Geometry: final body of the model. Coordinates: model frame, mm. A direction names the side the tool comes from. Coordinates: 2 decimals unless noted, no trailing zeros. Order: outer loops, then holes, each group sorted by start corner. A loop starts at its lowest first (then second) coordinate and runs counter-clockwise, first axis right, second up. Notation, with made-up numbers: M 66,-16 L 75,-16 A5 ccw 75,-8 Z; hole C -28.75,66 d9. An arc over 180 degrees is marked long. Use CSV: the item, a comma, the result in double quotes. Start each with the question number.
Q1. Section query C-C, the plane z = -38. Output: boundary loops of the cut face in (x, y), and give its area (3 significant figures).
Q2. Section query B-B, the plane x = 19.5. Output: boundary loops of the cut face in (y, z), and give its area (4 significant figures).
Q3. Mould query, pull axis Z, two halves, no side actions, for faces 1 (the face through (16, 25, -5)), 2 (the face through (-2, 0, -44)), 3 (the face through (10, 16, 50)), 4 (the face through (16, 25, -33)). Classes: +Z half, -Z half, draft (parallel to the pull), parting line (faces both ways), or undercut.
Q4. Section query D-D, the plane y = 3. Output: boundary loops of the cut face in (x, z), and give its area (3 significant figures).
Q5. First-contact query: P1, Ø4.5, axis at x = 9.5, z = 40, coming from the -Y side; P2, Ø0.9, axis at x = 2.5, z = -51.5, coming from the +Y side; P3, Ø7.5, axis at x = 12, y = 28, coming from the -Z side. Flat tips, straight axial feed; report the tip coordinate or a pass-through.
Q6. Access query for faces 5 (the face through (8.92, 25.31, -28.44)), 6 (the face through (12, 5.25, -43)), 7 (the face through (7, 14.75, 0)), 8 (the face through (7, 0.25, -51)), 9 (the face through (12, 7, -51)). Directions: +Z, -Z, +X, -X, +Y, -Y. A direction counts if a zero-diameter tool reaches every point of the face in a straight line with its end or side. Return the directions, or none.
Q7. Ray query, probe 1 along Z at (x, y) = (14.75, 23); probe 2 along Z at (x, y) = (15.5, 13.5); probe 3 along Z at (x, y) = (5.75, 8). Return the intervals inside material, ascending.
Q8. Section query A-A, the plane y = -7. Output: boundary loops of the cut face in (x, z).
from build123d import *

# Parameters (mm, degrees)
BOSS_EXTRUDE1_DEPTH      = 50
BOSS_EXTRUDE1_DEPTH_BACK = 50
CUT_EXTRUDE1_DEPTH       = 66.448930473
CUT_EXTRUDE1_DEPTH_BACK  = 66.448930473
SKETCH2_W                = 70
SKETCH2_H                = 29.5
SKETCH5_W                = 15
SKETCH5_H                = 9
CUT_EXTRUDE2_DEPTH       = 20
BOSS_EXTRUDE3_REACH      = 110.128
BOSS_EXTRUDE4_DEPTH      = 3


with BuildPart() as part:
    # Sketch1 → Boss-Extrude1 (new, two sides: drawn at the far end of the back side and taken through both)
    with BuildSketch(Plane.XY.offset(-BOSS_EXTRUDE1_DEPTH_BACK)):
        with BuildLine():
            Line((-2, -14.75), (2, -14.75))
            Line((2, -14.75), (2, 5.25))
            Line((2, 5.25), (22, 5.25))
            Line((22, 5.25), (22, 14.75))
            Line((22, 14.75), (22, 34.75))
            Line((22, 34.75), (10.449961479, 34.75))
            ThreePointArc((10.449961479, 34.75), (6.111442266, 23.465706156), (-2, 14.501190503))
            Line((-2, 14.501190503), (-2, -14.75))
        make_face()
    extrude(amount=BOSS_EXTRUDE1_DEPTH + BOSS_EXTRUDE1_DEPTH_BACK)

    # Sketch2 → Cut-Extrude1 (cut, two sides: drawn at the far end of the back side and taken through both)
    with BuildSketch(Plane(origin=(-2, 0, 0), x_dir=(0, 0, -1), z_dir=(1, 0, 0)).offset(-CUT_EXTRUDE1_DEPTH_BACK)):
        Rectangle(SKETCH2_W, SKETCH2_H)
    extrude(amount=CUT_EXTRUDE1_DEPTH + CUT_EXTRUDE1_DEPTH_BACK, mode=Mode.SUBTRACT)

    # Sketch5 → Cut-Extrude2 (cut)
    with BuildSketch(Plane(origin=(0, 34.75, 0), x_dir=(1, 0, 0), z_dir=(0, 1, 0))):
        with Locations((14.5, -28.5)):
            Rectangle(SKETCH5_W, SKETCH5_H)
        with Locations((14.5, -9.5)):
            Rectangle(SKETCH5_W, SKETCH5_H)
        with Locations((14.5, 9.5)):
            Rectangle(SKETCH5_W, SKETCH5_H)
        with Locations((14.5, 28.5)):
            Rectangle(SKETCH5_W, SKETCH5_H)
    extrude(amount=-CUT_EXTRUDE2_DEPTH, mode=Mode.SUBTRACT)

    # Boss-Extrude3: up to this face of the body (flat: up to its plane)
    boss_extrude3_end = Plane(part.part.faces().sort_by_distance((10.585369563, 14.996232635, -50))[0])
    # Sketch6 → Boss-Extrude3 (add, up to the picked face)
    with BuildSketch(Plane.XY.offset(50), mode=Mode.PRIVATE) as boss_extrude3_sk1:
        with BuildLine():
            Line((14.639320225, 34.75), (10.449961479, 34.75))
            ThreePointArc((10.449961479, 34.75), (9.109168973, 29.740022443), (7, 25.001984252))
            Line((7, 25.001984252), (7, 14.75))
            ThreePointArc((7, 14.75), (8.974829231, 25.454662693), (14.639320225, 34.75))
        make_face()
    boss_extrude3_tool1 = split(extrude(boss_extrude3_sk1.sketch, amount=-BOSS_EXTRUDE3_REACH, mode=Mode.PRIVATE), bisect_by=boss_extrude3_end, keep=Keep.BOTH, mode=Mode.PRIVATE)
    add(boss_extrude3_tool1.solids().sort_by(Axis((9.906803, 28.936431, 50), (0, 0, -1)))[0])

    # Sketch8 → Boss-Extrude4 (add)
    with BuildSketch(Plane(origin=(0, 0, -50), x_dir=(-1, 0, 0), z_dir=(0, 0, -1))):
        Polygon((-12, 0.25), (-2, 0.25), (-2, -14.75), (2, -14.75), (2, 14.501190503), (-12, 14.501190503), align=None)
    extrude(amount=BOSS_EXTRUDE4_DEPTH)


solid = part.part
Responses:
1,outline,"M -2,-14.75 L 2,-14.75 L 2,5.25 L 22,5.25 L 22,34.75 L 10.45,34.75 A33 cw -2,14.5 Z"
1,area,"627 mm²"
2,outline,"M 5.25,-50 L 34.75,-50 L 34.75,-33 L 14.75,-33 L 14.75,-35 L 5.25,-35 Z; M 5.25,35 L 14.75,35 L 14.75,33 L 34.75,33 L 34.75,50 L 5.25,50 Z; M 14.75,-24 L 34.75,-24 L 34.75,-14 L 14.75,-14 Z; M 14.75,-5 L 34.75,-5 L 34.75,5 L 14.75,5 Z; M 14.75,14 L 34.75,14 L 34.75,24 L 14.75,24 Z"
2,area,"1,565 mm²"
3,face 1,"undercut"
3,face 2,"draft"
3,face 3,"+Z half"
3,face 4,"undercut"
4,outline,"M -2,-53 L 12,-53 L 12,-50 L 2,-50 L 2,-35 L -2,-35 Z; M -2,35 L 2,35 L 2,50 L -2,50 Z"
4,area,"162 mm²"
5,P1,"stops at y = 5.25"
5,P2,"stops at y = 14.5"
5,P3,"stops at z = -50"
6,face 5,"+X, -Y"
6,face 6,"+Z, +X, -Y"
6,face 7,"+X, -X, -Y"
6,face 8,"+Z, -Z, +X, -Y"
6,face 9,"-Z, +X, +Y, -Y"
7,probe 1,"z = -50 to -33, -24 to -14, -5 to 5, 14 to 24, 33 to 50"
7,probe 2,"z = -50 to -35, 35 to 50"
7,probe 3,"z = -53 to -35, 35 to 50"
8,outline,"M -2,-53 L 2,-53 L 2,-35 L -2,-35 Z; M -2,35 L 2,35 L 2,50 L -2,50 Z"
